For this review, take the finished solid that the model builds, in its own axes (mm). Face numbers are marked on the shaded views. A direction names the side the tool comes from. Round coordinates to 2 decimals unless told otherwise and drop trailing zeros. Write each loop counter-clockwise with the first axis right and the second up, starting at its lowest first coordinate (ties: lowest second). Pieces come first, ordered by that corner, then holes.
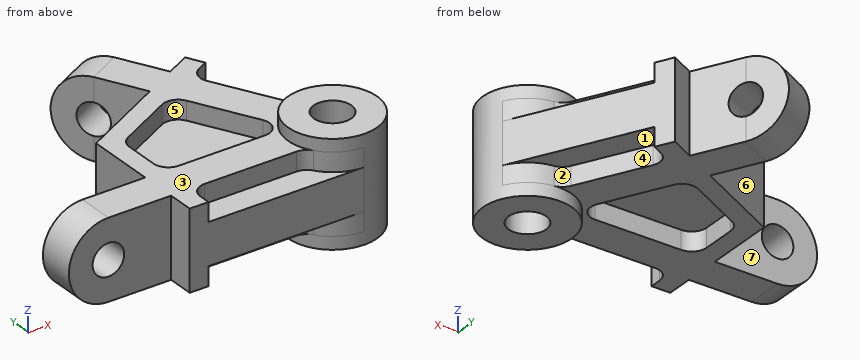
from build123d import *
from build123d.topology import SkipClean

# Parameters (mm, degrees)
BOSS_EXTRU_1_DEPTH      = 20
BOSS_EXTRU_2_DEPTH      = 26.35
BOSS_EXTRU_2_DEPTH_BACK = 26.35
ESQUISSE2_5_R           = 22.5
ESQUISSE2_5_R_2         = 9.5
BOSS_EXTRU_3_DEPTH      = 18.5
BOSS_EXTRU_4_DEPTH      = 18.5
ESQUISSE5_R             = 8
ENL_V_MAT_EXTRU_1_DEPTH = 188.483465609
ESQUISSE6_R             = 8
ENL_V_MAT_EXTRU_2_DEPTH = 190.711724403
ENL_V_START             = -9.5
ENL_V_MAT_EXTRU_3_DEPTH = 9.5


with BuildPart() as part:
    # Esquisse2 → Boss.-Extru.1 (new, symmetric)
    with BuildSketch(Plane.XY):
        with BuildLine():
            Line((-88.25, -22.5), (0, -22.5))
            ThreePointArc((0, -22.5), (-19.23551709, 11.672398309), (19.957743747, 10.389343798))
            Line((19.957743747, 10.389343798), (-16.981934979, 81.349806406))
            Line((-16.981934979, 81.349806406), (-28.734828519, 75.231637281))
            Line((-28.734828519, 75.231637281), (-40.740502796, 98.294322989))
            Line((-40.740502796, 98.294322989), (-57.15020321, 89.751973644))
            Line((-57.15020321, 89.751973644), (-45.144528933, 66.689287936))
            Line((-45.144528933, 66.689287936), (-88.25, 44.25))
            Line((-88.25, 44.25), (-88.25, 9.25))
            Line((-88.25, 9.25), (-120, 9.25))
            Line((-120, 9.25), (-120, -9.25))
            Line((-120, -9.25), (-88.25, -9.25))
            Line((-88.25, -9.25), (-88.25, -22.5))
        make_face()
    extrude(amount=BOSS_EXTRU_1_DEPTH, both=True)

    # Esquisse2<5> → Boss.-Extru.2 (add, two sides: drawn at the far end of the back side and taken through both)
    with BuildSketch(Plane.XY.offset(-BOSS_EXTRU_2_DEPTH_BACK)):
        Circle(ESQUISSE2_5_R)
        Circle(ESQUISSE2_5_R_2, mode=Mode.SUBTRACT)
    extrude(amount=BOSS_EXTRU_2_DEPTH + BOSS_EXTRU_2_DEPTH_BACK)

    # Esquisse3 → Boss.-Extru.3 (add)
    with BuildSketch(Plane.XZ.offset(9.25)):
        with BuildLine():
            Line((-120, 20), (-120, -20))
            ThreePointArc((-120, -20), (-140, 0), (-120, 20))
        make_face()
    extrude(amount=-BOSS_EXTRU_3_DEPTH)

    # Esquisse4 → Boss.-Extru.4 (add)
    with BuildSketch(Plane(origin=(8.204850207, 4.271174672, 0), x_dir=(0, 0, -1), z_dir=(0.8870108331782227, 0.46174861323503186, 0))):
        with BuildLine():
            Line((-20, 106), (20, 106))
            ThreePointArc((20, 106), (0, 126), (-20, 106))
        make_face()
    extrude(amount=-BOSS_EXTRU_4_DEPTH)

    # Esquisse5 → Enlèv. mat.-Extru.1 (cut, through all)
    with BuildSketch(Plane(origin=(8.204850207, 4.271174672, 0), x_dir=(0, 0, -1), z_dir=(0.8870108331782227, 0.46174861323503186, 0))):
        with Locations(Location((0, 106, 0), (0, 0, 90))):
            Circle(ESQUISSE5_R)
    extrude(amount=-ENL_V_MAT_EXTRU_1_DEPTH, mode=Mode.SUBTRACT)

    # Esquisse6 → Enlèv. mat.-Extru.2 (cut, through all)
    with BuildSketch(Plane.XZ.offset(9.25)):
        with Locations((-120, 0)):
            Circle(ESQUISSE6_R)
    extrude(amount=-ENL_V_MAT_EXTRU_2_DEPTH, mode=Mode.SUBTRACT)

    # Esquisse7 → Enlèv. mat.-Extru.3 (cut)
    with SkipClean():  # the faces are left unmerged after this step: merging them gives an invalid solid
        with BuildSketch(Plane.XY.offset(20).offset(ENL_V_START)):
            with BuildLine():
                Line((-17.695635444, 70.268148965), (-12.595323154, 72.923203491))
                Line((-12.595323154, 72.923203491), (19.957743747, 10.389343798))
                ThreePointArc((19.957743747, 10.389343798), (12.734529101, 18.549441193), (2.52390035, 22.3579947))
                ThreePointArc((2.52390035, 22.3579947), (-0.879642567, 23.627512536), (-3.287380782, 26.347545001))
                Line((-3.287380782, 26.347545001), (-20.885102094, 60.152453117))
                ThreePointArc((-20.885102094, 60.152453117), (-21.385397976, 65.870861212), (-17.695635444, 70.268148965))
            make_face()
            with BuildLine():
                Line((-74.713114599, 40.586728011), (-47.410498356, 54.799570422))
                ThreePointArc((-47.410498356, 54.799570422), (-41.69209026, 55.299866303), (-37.294802508, 51.610103772))
                Line((-37.294802508, 51.610103772), (-20.950564458, 20.213114599))
                ThreePointArc((-20.950564458, 20.213114599), (-21.191306677, 12.859200564), (-27.603145707, 9.25))
                Line((-27.603145707, 9.25), (-71.25, 9.25))
                ThreePointArc((-71.25, 9.25), (-76.553300859, 11.446699141), (-78.75, 16.75))
                Line((-78.75, 16.75), (-78.75, 33.934146763))
                ThreePointArc((-78.75, 33.934146763), (-77.66183903, 37.824946199), (-74.713114599, 40.586728011))
            make_face()
            with BuildLine():
                Line((-71.25, -9.25), (-24.888501361, -9.25))
                ThreePointArc((-24.888501361, -9.25), (-21.364033316, -10.129718662), (-18.666376021, -12.5625))
                ThreePointArc((-18.666376021, -12.5625), (-10.573404135, -19.860844015), (0, -22.5))
                Line((0, -22.5), (-78.75, -22.5))
                Line((-78.75, -22.5), (-78.75, -16.75))
                ThreePointArc((-78.75, -16.75), (-76.553300859, -11.446699141), (-71.25, -9.25))
            make_face()
        enl_v_mat_extru_3 = extrude(amount=ENL_V_MAT_EXTRU_3_DEPTH, mode=Mode.SUBTRACT)

    # Symétrie1: Enlèv. mat.-Extru.3 across plane
    add(enl_v_mat_extru_3.mirror(Plane.XY), mode=Mode.SUBTRACT)


solid = part.part
(1) We need section A-A, the plane y = 0. Give the boundary of the cut face in (x, z), and give its area (3 significant figures).
Geometry check:
outline: (-120, -20) - (-22.5, -20) - (-22.5, -26.35) - (-9.5, -26.35) - (-9.5, 26.35) - (-22.5, 26.35) - (-22.5, 20) - (-120, 20) arc R20 ccw to start; (9.5, -26.35) - (22.5, -26.35) - (22.5, 26.35) - (9.5, 26.35) - close; hole circle Ø16 at (-120, 0)
area: 5,700 mm2
(2) For line 1 along Z through (x, y) = (-120, 5.5); line 2 along X through (y, z) = (-8, -3.5); line 3 along Z through (x, y) = (-80.5, 35), list the stretches that pass through material, from the lowest coordinate up.
Geometry check:
line 1: z = -20 to -8, 8 to 20
line 2: x = -139.69 to -127.19, -112.81 to -5.12, 5.12 to 21.03
line 3: z = -20 to 20
(3) For pin 1 Ø8 at (x, z) = (-59.5, 5.5) entering from +Y; pin 2 Ø6.5 at (x, y) = (-37.5, -14) entering from -Z; pin 3 Ø5 at (y, z) = (73, -19.5) entering from +X; pin 4 Ø17 at (x, y) = (0, 0) entering from -Z, all flat-tipped, find the tip position at first contact; note any pin that passes through.
Geometry check:
pin 1: stops at y = 112.55
pin 2: stops at z = -10.5
pin 3: stops at x = -12.6
pin 4: passes through
(4) Mouldability with a two-part tool opening along Y and no side actions: class the marked faces 1, 2 and 3 as pulls with the +Y half, pulls with the -Y half, needs draft (parallel to the pull), parting line crosses it, or undercut.
Geometry check:
face 1: undercut
face 2: pulls with the +Y half
face 3: needs draft
(5) For the marked faces 4, 5, 6 and 7, list the 3-axis set-ups (+Z, -Z, +X, -X, +Y, -Y) from which the entire face can be reached by the end or side of a thin tool; tool diameter is ignored.
Geometry check:
face 4: -Z, +X
face 5: +Z
face 6: +Z, -Z, -X
face 7: +Z, -Z, -X, +Y
(6) We need section B-B, the plane z = 5. Give the boundary of the cut face in (x, y) (3 decimals), and give its area (3 significant figures).
Geometry check:
outline: (-139.365, -9.25) - (-126.245, -9.25) - (-126.245, 9.25) - (-139.365, 9.25) - close; (-113.755, -9.25) - (-88.25, -9.25) - (-88.25, -22.5) - (0, -22.5) arc R22.5 ccw to (19.958, 10.389) - (-16.982, 81.35) - (-28.735, 75.232) - (-37.857, 92.755) - (-54.267, 84.213) - (-45.145, 66.689) - (-88.25, 44.25) - (-88.25, 9.25) - (-113.755, 9.25) - close; (-66.092, 106.929) - (-60.034, 95.291) - (-43.624, 103.834) - (-49.682, 115.471) - close; hole circle Ø19 at (0, 0)
area: 9,610 mm2
(7) We need section C-C, the plane x = 5.5. Give the boundary of the cut face in (y, z).
Geometry check:
outline: (-21.82, -26.35) - (-7.75, -26.35) - (-7.75, 26.35) - (-21.82, 26.35) - close; (7.75, -26.35) - (21.82, -26.35) - (21.82, -10.5) - (38.16, -10.5) - (38.16, 10.5) - (21.82, 10.5) - (21.82, 26.35) - (7.75, 26.35) - close
(8) We need section D-D, the plane z = 14. State how many separate pieces and enclosed holes the cut face has, and give its area (3 significant figures).
Geometry check:
separate pieces: 1
enclosed holes: 2
area: 6,280 mm2
